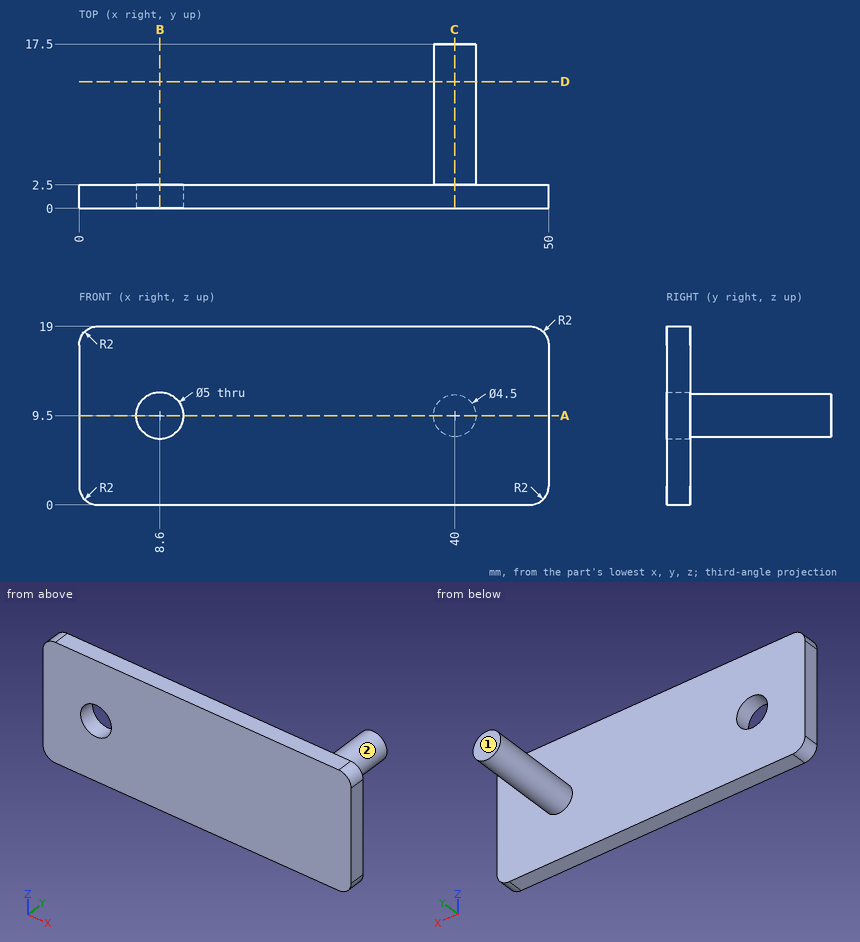
Verification items for this drawing (mm, ordinates from the low corner). A direction names the side the tool comes from. Coordinates: 2 decimals unless noted, no trailing zeros. Order: outer loops, then holes, each group sorted by start corner. A loop starts at its lowest first (then second) coordinate and runs counter-clockwise, first axis right, second up. Notation, with made-up numbers: (54, 12.25) - (77, 12.25) arc R13 ccw to (77, 21.25) - close; hole circle Ø8 at (4, 43). An arc over 180 degrees is marked (long way). Answer in a Markdown table with one row per item. Add a question column.
1. Gauge pin test, flat ends, axial feed: pin 1 Ø10 at (x, y) = (40.5, 3.5) entering from -Z; pin 2 Ø5 at (x, z) = (7.5, 11.5) entering from +Y; pin 3 Ø4 at (y, z) = (9, 5.5) entering from -X; pin 4 Ø6 at (y, z) = (6.5, 2) entering from +X. Record the tip position at first contact, or that the pin passes through.
2. Material ranges on L1, parallel to X at y = 1.3, z = 9.5; L2, parallel to Y at x = 40, z = 3.5; L3, parallel to X at y = 8.25, z = 8.75, recorded low to high. Write a range as [from, to].
3. Section check A-A (z = 9.5). Enter the section's corners in (x, y).
4. Section check D-D (y = 13.5). Enter the section's corners in (x, z), plus the area to 3 significant figures.
5. Section check C-C (x = 40). Enter the section's corners in (y, z), plus the area to 3 significant figures.
6. Section check B-B (x = 8.6). Enter the section's corners in (y, z), plus the area to 3 significant figures.
7. Access from +Z, -Z, +X, -X, +Y, -Y to the whole of each face (thin tool, end or side, straight path). Record for the marked faces 1 and 2.
Data:
| question | item | result |
|---|---|---|
| 1 | pin 1 | stops at z = 0 |
| 1 | pin 2 | stops at y = 2.5 |
| 1 | pin 3 | stops at x = 38.97 |
| 1 | pin 4 | passes through |
| 2 | L1 | x = [0, 6.1], [11.1, 50] |
| 2 | L2 | y = [0, 2.5] |
| 2 | L3 | x = [37.88, 42.12] |
| 3 | outline | (0, 0) - (6.1, 0) - (6.1, 2.5) - (0, 2.5) - close; (11.1, 0) - (50, 0) - (50, 2.5) - (42.25, 2.5) - (42.25, 17.5) - (37.75, 17.5) - (37.75, 2.5) - (11.1, 2.5) - close |
| 4 | outline | circle Ø4.5 at (40, 9.5) |
| 4 | area | 15.9 mm² |
| 5 | outline | (0, 0) - (2.5, 0) - (2.5, 7.25) - (17.5, 7.25) - (17.5, 11.75) - (2.5, 11.75) - (2.5, 19) - (0, 19) - close |
| 5 | area | 115 mm² |
| 6 | outline | (0, 0) - (2.5, 0) - (2.5, 7) - (0, 7) - close; (0, 12) - (2.5, 12) - (2.5, 19) - (0, 19) - close |
| 6 | area | 35.0 mm² |
| 7 | face 1 | +Z, -Z, +X, -X, +Y |
| 7 | face 2 | +Y |
